```python
from build123d import *

# Parameters (mm, degrees)
SKETCH1_W           = 6.666666666
SKETCH1_H           = 40
BOSS_EXTRUDE1_DEPTH = 0.5
SKETCH1_3_W         = 1
SKETCH1_3_H         = 40
BOSS_EXTRUDE2_DEPTH = 6.23
SKETCH2_W           = 1
SKETCH2_H           = 0.5
BOSS_EXTRUDE3_DEPTH = 2
SKETCH3_W           = 1
SKETCH3_H           = 0.5
BOSS_EXTRUDE4_DEPTH = 0.5
CUT_EXTRUDE1_DEPTH  = 43.680096975
CUT_EXTRUDE2_DEPTH  = 24.143264199


with BuildPart() as part:
    # Sketch1 → Boss-Extrude1 (new body)
    with BuildSketch(Plane(origin=(0, 0, 0), x_dir=(1, 0, 0), z_dir=(0, 1, 0))):
        Rectangle(SKETCH1_W, SKETCH1_H)
    extrude(amount=BOSS_EXTRUDE1_DEPTH)

    # Sketch1<3> → Boss-Extrude2 (add)
    with BuildSketch(Plane(origin=(0, 0, 0), x_dir=(1, 0, 0), z_dir=(0, 1, 0))):
        with Locations((-3.833333333, 0)):
            Rectangle(SKETCH1_3_W, SKETCH1_3_H)
        with Locations((3.833333333, 0)):
            Rectangle(SKETCH1_3_W, SKETCH1_3_H)
    extrude(amount=BOSS_EXTRUDE2_DEPTH)

    # Sketch2 → Boss-Extrude3 (add)
    with BuildSketch(Plane.XY.offset(20)):
        with Locations((-3.833333333, 0.75)):
            Rectangle(SKETCH2_W, SKETCH2_H)
        with Locations((3.833333333, 0.75)):
            Rectangle(SKETCH2_W, SKETCH2_H)
    boss_extrude3 = extrude(amount=BOSS_EXTRUDE3_DEPTH)

    # Sketch3 → Boss-Extrude4 (add)
    with BuildSketch(Plane.XZ.offset(-0.5)):
        with Locations((-3.833333333, 21.75)):
            Rectangle(SKETCH3_W, SKETCH3_H)
        with Locations((3.833333333, 21.75)):
            Rectangle(SKETCH3_W, SKETCH3_H)
    boss_extrude4 = extrude(amount=BOSS_EXTRUDE4_DEPTH)

    # Mirror1: Boss-Extrude3, Boss-Extrude4 across plane
    add(boss_extrude3.mirror(Plane.XY))
    add(boss_extrude4.mirror(Plane.XY))

    # Sketch5 → Cut-Extrude1 (cut, through all)
    with BuildSketch(Plane.XY.offset(20)):
        with BuildLine():
            Line((-4.333333333, 6.23), (-4.333333333, 5.73))
            ThreePointArc((-4.333333333, 5.73), (-4.186886724, 6.083553391), (-3.833333333, 6.23))
            Line((-3.833333333, 6.23), (-4.333333333, 6.23))
        make_face()
        with BuildLine():
            Line((-3.333333333, 6.23), (-3.833333333, 6.23))
            ThreePointArc((-3.833333333, 6.23), (-3.479779943, 6.083553391), (-3.333333333, 5.73))
            Line((-3.333333333, 5.73), (-3.333333333, 6.23))
        make_face()
        with BuildLine():
            Line((3.833333333, 6.23), (3.333333333, 6.23))
            Line((3.333333333, 6.23), (3.333333333, 5.73))
            ThreePointArc((3.333333333, 5.73), (3.479779943, 6.083553391), (3.833333333, 6.23))
        make_face()
        with BuildLine():
            Line((4.333333333, 6.23), (3.833333333, 6.23))
            ThreePointArc((3.833333333, 6.23), (4.186886724, 6.083553391), (4.333333333, 5.73))
            Line((4.333333333, 5.73), (4.333333333, 6.23))
        make_face()
    extrude(amount=-CUT_EXTRUDE1_DEPTH, mode=Mode.SUBTRACT)

    # Sketch6 → Cut-Extrude2 (cut, through all)
    with BuildSketch(Plane(origin=(0, 0.5, 0), x_dir=(1, 0, 0), z_dir=(0, 1, 0))):
        with BuildLine():
            Line((2.13569746, 4.561085027), (2.13569746, -4.561085027))
            ThreePointArc((2.13569746, -4.561085027), (0, -6.696782487), (-2.13569746, -4.561085027))
            Line((-2.13569746, -4.561085027), (-2.13569746, 4.561085027))
            ThreePointArc((-2.13569746, 4.561085027), (0, 6.696782487), (2.13569746, 4.561085027))
        make_face()
        with BuildLine():
            Line((2.13569746, 24.862478311), (2.13569746, 15.137521689))
            ThreePointArc((2.13569746, 15.137521689), (0, 13.001824229), (-2.13569746, 15.137521689))
            Line((-2.13569746, 15.137521689), (-2.13569746, 24.862478311))
            ThreePointArc((-2.13569746, 24.862478311), (0, 26.998175771), (2.13569746, 24.862478311))
        make_face()
        with BuildLine():
            Line((2.13569746, -24.862478311), (2.13569746, -15.137521689))
            ThreePointArc((2.13569746, -15.137521689), (0, -13.001824229), (-2.13569746, -15.137521689))
            Line((-2.13569746, -15.137521689), (-2.13569746, -24.862478311))
            ThreePointArc((-2.13569746, -24.862478311), (0, -26.998175771), (2.13569746, -24.862478311))
        make_face()
    extrude(amount=-CUT_EXTRUDE2_DEPTH, mode=Mode.SUBTRACT)


solid = part.part
```
Build history of the part. All positions in model axes, mm. A direction names the side the tool comes from. Coordinates: 2 decimals unless noted, no trailing zeros. Write each loop counter-clockwise with the first axis right and the second up, starting at its lowest first coordinate (ties: lowest second). Pieces come first, ordered by that corner, then holes.
1. Drill centre lines: probe 1 along X at (y, z) = (4, 8); probe 2 along Z at (x, y) = (-4, 4.5); probe 3 along Y at (x, z) = (3, 5.5). Where is each one in solid material? Low to high.
Answer block:
probe 1: x = -4.33 to -3.33, 3.33 to 4.33
probe 2: z = -20 to 20
probe 3: y = 0 to 0.5
2. Pull direction Z, two halves, no side cores. Call faces 1 (the cylindrical face through (0, 0.3, 13)), 2 (the flat face through (-4, 0.5, 21)), 3 (the flat face through (-4, 1, 21)): released by +Z, released by -Z, zero draft, split by the parting line, or undercut.
Answer block:
face 1: released by +Z
face 2: undercut
face 3: zero draft
3. Band-saw the part on A-A, the plane x = 0. Give the cut face in (y, z).
Answer block:
outline: (0, -13) - (0.5, -13) - (0.5, -6.7) - (0, -6.7) - close; (0, 6.7) - (0.5, 6.7) - (0.5, 13) - (0, 13) - close
4. Drop flat-ended pins along their axis: pin 1 (0.5 mm diameter, centred on x = -4, z = 21, fed in from +Y); pin 2 (1.5 mm diameter, centred on x = 2, y = 3, fed in from +Z); pin 3 (0.8 mm diameter, centred on x = 3.5, y = 2.5, fed in from +Z); pin 4 (1.1 mm diameter, centred on x = 4, y = 4, fed in from -Z). Give the stop position or say it passes through.
Answer block:
pin 1: stops at y = 1
pin 2: passes through
pin 3: stops at z = 20
pin 4: stops at z = -20
5. Band-saw the part on D-D, the plane z = -9.5. Give the cut face in (x, y), and give its area (3 significant figures).
Answer block:
outline: (-4.33, 0) - (4.33, 0) - (4.33, 5.73) arc R0.5 ccw to (3.33, 5.73) - (3.33, 0.5) - (-3.33, 0.5) - (-3.33, 5.73) arc R0.5 ccw to (-4.33, 5.73) - close
area: 15.6 mm2
6. 3-axis set-ups, long thin cutter, end or side, ignore diameter. For faces 4 (the flat face through (3, 0, 0)), 5 (the cylindrical face through (-0.047, 0.254, -6.696)), 6 (the flat face through (-4, 4, 20)), 7 (the flat face through (4, 0.5, 21)), 8 (the flat face through (4, 1, -21)): which of +Z, -Z, +X, -X, +Y, -Y reach the whole face in a straight line?
Answer block:
face 4: +Z, -Z, +X, -X, -Y
face 5: +Y, -Y
face 6: +Z, +X, -X, +Y
face 7: +X, -X, -Y
face 8: -Z, +X, -X, +Y
7. Band-saw the part on C-C, the plane z = -17. Give the cut face in (x, y).
Answer block:
outline: (-4.33, 0) - (-2.14, 0) - (-2.14, 0.5) - (-3.33, 0.5) - (-3.33, 5.73) arc R0.5 ccw to (-4.33, 5.73) - close; (2.14, 0) - (4.33, 0) - (4.33, 5.73) arc R0.5 ccw to (3.33, 5.73) - (3.33, 0.5) - (2.14, 0.5) - close
8. Band-saw the part on B-B, the plane y = 1.5. Give the cut face in (x, z).
Answer block:
outline: (-4.33, -20) - (-3.33, -20) - (-3.33, 20) - (-4.33, 20) - close; (3.33, -20) - (4.33, -20) - (4.33, 20) - (3.33, 20) - close
